from build123d import *

# Parameters (mm, degrees)
SKETCH1_W           = 120
SKETCH1_H           = 45
SKETCH1_R           = 11.3625
SKETCH1_R_2         = 1.65
BOSS_EXTRUDE1_DEPTH = 6
CUT_EXTRUDE1_START  = -6
SKETCH2_R           = 3
SKETCH2_R_2         = 1.65
CUT_EXTRUDE1_DEPTH  = 3


with BuildPart() as part:
    # Sketch1 → Boss-Extrude1 (new body)
    with BuildSketch(Plane.XY):
        with Locations((60, 22.5)):
            Rectangle(SKETCH1_W, SKETCH1_H)
        with Locations((64, 30)):
            Circle(SKETCH1_R, mode=Mode.SUBTRACT)
        with Locations((4, 41)):
            Circle(SKETCH1_R_2, mode=Mode.SUBTRACT)
        with Locations(Location((4, 4, 0), (0, 0, 180))):
            Circle(SKETCH1_R_2, mode=Mode.SUBTRACT)
        with Locations(Location((116, 41, 0), (0, 0, 180))):
            Circle(SKETCH1_R_2, mode=Mode.SUBTRACT)
        with Locations((116, 4)):
            Circle(SKETCH1_R_2, mode=Mode.SUBTRACT)
    extrude(amount=BOSS_EXTRUDE1_DEPTH)

    # Sketch2 → Cut-Extrude1 (cut)
    # profile 1 of 4: a face of its own
    with BuildSketch(Plane.XY.offset(6).offset(CUT_EXTRUDE1_START)):
        with Locations(Location((4, 41, 0), (0, 0, 180))):
            Circle(SKETCH2_R)
        with Locations(Location((4, 41, 0), (0, 0, 180))):
            Circle(SKETCH2_R_2, mode=Mode.SUBTRACT)
    # profile 2 of 4: a face of its own
    with BuildSketch(Plane.XY.offset(6).offset(CUT_EXTRUDE1_START)):
        with Locations(Location((4, 4, 0), (0, 0, 180))):
            Circle(SKETCH2_R)
        with Locations(Location((4, 4, 0), (0, 0, 180))):
            Circle(SKETCH2_R_2, mode=Mode.SUBTRACT)
    # profile 3 of 4: a face of its own
    with BuildSketch(Plane.XY.offset(6).offset(CUT_EXTRUDE1_START)):
        with Locations(Location((116, 4, 0), (0, 0, 180))):
            Circle(SKETCH2_R)
        with Locations(Location((116, 4, 0), (0, 0, 180))):
            Circle(SKETCH2_R_2, mode=Mode.SUBTRACT)
    # profile 4 of 4: a face of its own
    with BuildSketch(Plane.XY.offset(6).offset(CUT_EXTRUDE1_START)):
        with Locations(Location((116, 41, 0), (0, 0, 180))):
            Circle(SKETCH2_R)
        with Locations(Location((116, 41, 0), (0, 0, 180))):
            Circle(SKETCH2_R_2, mode=Mode.SUBTRACT)
    extrude(amount=CUT_EXTRUDE1_DEPTH, mode=Mode.SUBTRACT)


solid = part.part
Read the model definition and answer for the solid it produces. Units are mm, in the model's axes. A direction names the side the tool comes from. Give positions to 0.01 mm unless a question says otherwise; leave off trailing zeros. Loops run counter-clockwise (first coordinate to the right, second up) from the corner with the lowest first, then second, coordinate; pieces in that order, holes last. Notation, with made-up numbers: M -27.75,58.25 L 15.25,58.25 A22 ccw 15.25,67.25 Z; hole C -36.75,-4.75 d2. An arc over 180 degrees is marked long. Write each question's results on one line, items separated by ' | '.
1. Section B-B on x = 116 is taken. Give the vertices of the cut face in (y, z), plus the area to 3 significant figures.
Values:
outline: M 0,0 L 1,0 L 1,3 L 2.35,3 L 2.35,6 L 0,6 Z; M 5.65,3 L 7,3 L 7,0 L 38,0 L 38,3 L 39.35,3 L 39.35,6 L 5.65,6 Z; M 42.65,3 L 44,3 L 44,0 L 45,0 L 45,6 L 42.65,6 Z | area: 214 mm^2
2. Given pin 1 (3 mm diameter, centred on x = 117, y = 5, fed in from -Z); pin 2 (20.5 mm diameter, centred on x = 64, y = 30, fed in from +Z), each flat-ended and moving along its own axis, determine where each tip first touches the part or whether it passes through.
Values:
pin 1: stops at z = 3 | pin 2: passes through
3. The mould has two halves that part along X. Classify faces 3 (the face through (59, 18, 0)), 4 (the face through (0, 22, 3)), 5 (the face through (117.524, 3.368, 4.479)): pulls with the +X half, pulls with the -X half, needs draft (parallel to the pull), parting line crosses it, or undercut.
Values:
face 3: needs draft | face 4: pulls with the -X half | face 5: undercut
4. Section D-D on z = 4.3 is taken. State how many separate pieces and enclosed holes the cut face has, plus the area to 3 significant figures.
Values:
separate pieces: 1 | enclosed holes: 5 | area: 4,960 mm^2
5. Section A-A on y = 4 is taken. Give the vertices of the cut face in (x, z).
Values:
outline: M 0,0 L 1,0 L 1,3 L 2.35,3 L 2.35,6 L 0,6 Z; M 5.65,3 L 7,3 L 7,0 L 113,0 L 113,3 L 114.35,3 L 114.35,6 L 5.65,6 Z; M 117.65,3 L 119,3 L 119,0 L 120,0 L 120,6 L 117.65,6 Z
6. A tool of negligible diameter and unlimited length cuts with its end or side. For faces 1 (the face through (113.14, 40.1, 1.48)), 2 (the face through (54.98, 23.09, 2.96)), from which of +Z, -Z, +X, -X, +Y, -Y can it reach the whole face along a straight path? Write none if from no direction.
Values:
face 1: -Z | face 2: +Z, -Z
7. Section C-C on y = 30 is taken. Give the vertices of the cut face in (x, z), plus the area to 3 significant figures.
Values:
outline: M 0,0 L 52.64,0 L 52.64,6 L 0,6 Z; M 75.36,0 L 120,0 L 120,6 L 75.36,6 Z | area: 584 mm^2
8. Straight lines are drawn through the part: line 1 (Y direction, x = 4, z = 5.3); line 2 (X direction, y = 4, z = 1.95); line 3 (Y direction, x = 116, z = 1.85). For each, find the intervals that lie inside material, in ascending order. Write a range as [from, to].
Values:
line 1: y = [0, 2.35], [5.65, 39.35], [42.65, 45] | line 2: x = [0, 1], [7, 113], [119, 120] | line 3: y = [0, 1], [7, 38], [44, 45]
